The model under review builds one solid part; all positions refer to its coordinate system, in mm. Face numbers are marked on the shaded views. A direction names the side the tool comes from. Round coordinates to 2 decimals unless told otherwise and drop trailing zeros. Return JSON: item names as keys, results as strings. Group by question number.
1. Tool access review of the marked faces 1 and 2: name each direction out of +Z, -Z, +X, -X, +Y, -Y from which nothing blocks a thin tool from reaching the whole face with its end or side.
2. For line 1 along Y through (x, z) = (0, 21.25); line 2 along X through (y, z) = (-7, 25); line 3 along Y through (x, z) = (0, 24), list the stretches that pass through material, from the lowest coordinate up. Write a range as from..to.
3. Clearance check with flat-ended pins moving along their axes: P1, Ø1, axis at x = 22.5, z = -29.5, coming from the -Y side; P2, Ø1, axis at x = -8.5, z = 19, coming from the -Y side; P3, Ø3, axis at x = 11, y = 13.5, coming from the +Z side. State where each tip first meets the part, or that it passes through.
from build123d import *

# Parameters (mm, degrees)
F2_SIZE  = 5.08
F4_R     = 19.05
F5_DEPTH = 11.43


with BuildPart() as f1:
    # F0 (on Front) → F1 (revolve)
    with BuildSketch(Plane.XZ):
        Polygon((0, -17.9517306387), (0, 30.058646322), (-22.86, 30.058646322), (-38.1891950965, -39.389681071), (-0.0891950965, -39.389681071), align=None)
    revolve(axis=Axis((-0.0445975482, 0, -28.6707058549), (-0.0041605808, 0, -0.9999913447)))

    # F2
    f2_edges = [f1.edges().sort_by_distance(p)[0] for p in [
        (23.258707, 0, 29.866764),
    ]]
    chamfer(f2_edges, length=F2_SIZE)

    # F4 (on offset) → F5 (cut)
    with BuildSketch(Plane.XY.offset(30.0736)):
        Circle(F4_R)
    extrude(amount=-F5_DEPTH, mode=Mode.SUBTRACT)


solid = f1.part
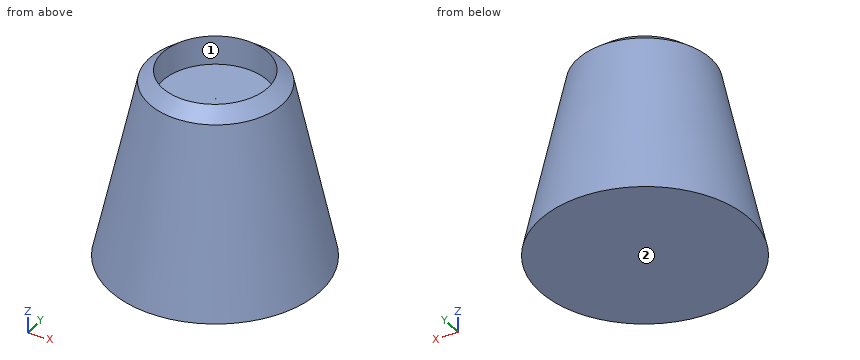
Output:
{
 "1": {"face 1": "+Z", "face 2": "-Z, -X"},
 "2": {"line 1": "y = -24.94..-19.05, 19.05..24.94", "line 2": "x = -22.94..-17.72, 17.72..23.15", "line 3": "y = -24.35..-19.05, 19.05..24.35"},
 "3": {"P1": "stops at y = -28.36", "P2": "stops at y = -24.13", "P3": "stops at z = 18.64"}
}
